Part model, mm, in its own coordinate system. Face numbers are marked on the shaded views. A direction names the side the tool comes from. Give positions to 0.01 mm unless a question says otherwise; leave off trailing zeros. Loops run counter-clockwise (first coordinate to the right, second up) from the corner with the lowest first, then second, coordinate; pieces in that order, holes last. Notation, with made-up numbers: M 43,-12.5 L 59,-12.5 A17 cw 59,10.5 Z; hole C -37.75,17.5 d8. An arc over 180 degrees is marked long. Put each result on its own line as item: value. Start each with the question number.
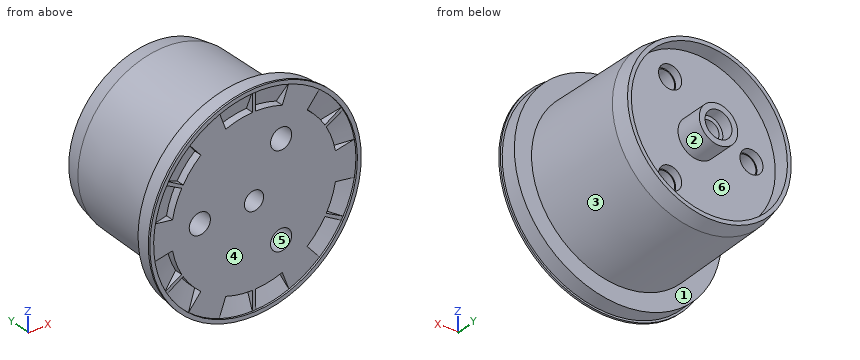
```python
from build123d import *

# Parameters (mm, degrees)
SCHIZZO1_R                    = 22
ESTRUSIONE_ESTRUSIONE1_DEPTH  = 30
SFORMO1_ANGLE                 = 1
SMUSSO1_SIZE                  = 4
SMUSSO1_SIZE2                 = 0.707593191
SCHIZZO2_R                    = 20.292406809
TAGLIO_ESTRUSIONE1_DEPTH      = 4
SCHIZZO4_R                    = 3
TAGLIO_ESTRUSIONE2_DEPTH      = 2
SCHIZZO3_R                    = 5
ESTRUSIONE_ESTRUSIONE2_DEPTH  = 7
SCHIZZO6_R                    = 3.5
TAGLIO_ESTRUSIONE5_DEPTH      = 3
SCHIZZO14_R                   = 27
SCHIZZO14_R_2                 = 22.5
ESTRUSIONE_ESTRUSIONE8_DEPTH  = 4
SCHIZZO16_R                   = 27.5
SCHIZZO16_R_2                 = 26.5
ESTRUSIONE_ESTRUSIONE9_DEPTH  = 0.5
SCHIZZO21_R                   = 22.5
ESTRUSIONE_ESTRUSIONE12_DEPTH = 4
SCHIZZO5_R                    = 2.75
TAGLIO_ESTRUSIONE3_DEPTH      = 49.215661356
RIPETIZIONECIRCOLARE1_COUNT   = 3
SCHIZZO24_R                   = 2.5
TAGLIO_ESTRUSIONE11_DEPTH     = 52.98797938
TAGLIA_RIVOLUZIONE1_ANGLE     = 40
RIVOLUZIONE1_ANGLE            = 2
RIPETIZIONECIRCOLARE2_COUNT   = 6


# Read off the part's stored shape, not the designer's step: Taglia-Rivoluzione1
with BuildPart() as part:
    # Schizzo1 → Estrusione-Estrusione1 (new body)
    with BuildSketch(Plane(origin=(0, 0, 0), x_dir=(1, 0, 0), z_dir=(0, 1, 0))):
        with Locations(Location((0, 0, 0), (0, 0, 270))):
            Circle(SCHIZZO1_R)
    extrude(amount=ESTRUSIONE_ESTRUSIONE1_DEPTH)

    # Sformo1
    sformo1_faces = [part.faces().sort_by_distance(p)[0] for p in [
        (0, 15, -22),
    ]]
    draft(sformo1_faces, Plane.ZX.offset(30), SFORMO1_ANGLE)

    # Smusso1
    smusso1_edges = [part.edges().sort_by_distance(p)[0] for p in [
        (0, 30, -22),
    ]]
    smusso1_side = [part.faces().sort_by_distance(p)[0] for p in [
        (0, 15, -22.261825974),
    ]]
    chamfer(smusso1_edges, length=SMUSSO1_SIZE, length2=SMUSSO1_SIZE2, reference=smusso1_side[0])

    # Schizzo2 → Taglio-Estrusione1 (cut)
    with BuildSketch(Plane(origin=(0, 30, 0), x_dir=(1, 0, 0), z_dir=(0, 1, 0))):
        with Locations(Location((0, 0, 0), (0, 0, 270))):
            Circle(SCHIZZO2_R)
    extrude(amount=-TAGLIO_ESTRUSIONE1_DEPTH, mode=Mode.SUBTRACT)

    # Schizzo4 → Taglio-Estrusione2 (cut)
    with BuildSketch(Plane(origin=(0, 26, 0), x_dir=(1, 0, 0), z_dir=(0, 1, 0))):
        with Locations(Location((7.05, 12.210958193, 0), (0, 0, 270))):
            Circle(SCHIZZO4_R)
    taglio_estrusione2 = extrude(amount=-TAGLIO_ESTRUSIONE2_DEPTH, mode=Mode.SUBTRACT)

    # Schizzo3 → Estrusione-Estrusione2 (add)
    with BuildSketch(Plane(origin=(0, 26, 0), x_dir=(1, 0, 0), z_dir=(0, 1, 0))):
        with Locations(Location((0, 0, 0), (0, 0, 270))):
            Circle(SCHIZZO3_R)
    extrude(amount=ESTRUSIONE_ESTRUSIONE2_DEPTH)

    # Schizzo6 → Taglio-Estrusione5 (cut)
    with BuildSketch(Plane(origin=(0, 33, 0), x_dir=(1, 0, 0), z_dir=(0, 1, 0))):
        with Locations(Location((0, 0, 0), (0, 0, 270))):
            Circle(SCHIZZO6_R)
    extrude(amount=-TAGLIO_ESTRUSIONE5_DEPTH, mode=Mode.SUBTRACT)

    # Schizzo14 → Estrusione-Estrusione8 (add)
    with BuildSketch(Plane.XZ):
        with Locations(Location((0, 0, 0), (0, 0, 270))):
            Circle(SCHIZZO14_R)
        with Locations(Location((0, 0, 0), (0, 0, 270))):
            Circle(SCHIZZO14_R_2, mode=Mode.SUBTRACT)
    extrude(amount=ESTRUSIONE_ESTRUSIONE8_DEPTH)

    # Schizzo16 → Estrusione-Estrusione9 (add)
    with BuildSketch(Plane.XZ.offset(4)):
        with Locations(Location((0, 0, 0), (0, 0, 270))):
            Circle(SCHIZZO16_R)
        with Locations(Location((0, 0, 0), (0, 0, 270))):
            Circle(SCHIZZO16_R_2, mode=Mode.SUBTRACT)
    extrude(amount=ESTRUSIONE_ESTRUSIONE9_DEPTH)

    # Schizzo21 → Estrusione-Estrusione12 (add)
    with BuildSketch(Plane.XZ):
        Circle(SCHIZZO21_R)
    extrude(amount=ESTRUSIONE_ESTRUSIONE12_DEPTH)

    # Schizzo5 → Taglio-Estrusione3 (cut, symmetric)
    with BuildSketch(Plane(origin=(0, 24, 0), x_dir=(1, 0, 0), z_dir=(0, 1, 0))):
        with Locations(Location((7.05, 12.210958193, 0), (0, 0, 270))):
            Circle(SCHIZZO5_R)
    taglio_estrusione3 = extrude(amount=TAGLIO_ESTRUSIONE3_DEPTH, both=True, mode=Mode.SUBTRACT)

    # RipetizioneCircolare1: Taglio-Estrusione2, Taglio-Estrusione3 ×3 about axis
    ripetizionecircolare1_axis = Axis((0, 0, 0), (0, 1, 0))
    add([taglio_estrusione2.rotate(ripetizionecircolare1_axis, i * 360 / RIPETIZIONECIRCOLARE1_COUNT) for i in range(1, RIPETIZIONECIRCOLARE1_COUNT)], mode=Mode.SUBTRACT)
    add([taglio_estrusione3.rotate(ripetizionecircolare1_axis, i * 360 / RIPETIZIONECIRCOLARE1_COUNT) for i in range(1, RIPETIZIONECIRCOLARE1_COUNT)], mode=Mode.SUBTRACT)

    # Schizzo24 → Taglio-Estrusione11 (cut, through all)
    with BuildSketch(Plane(origin=(0, 30, 0), x_dir=(1, 0, 0), z_dir=(0, 1, 0))):
        with Locations(Location((0, 0, 0), (0, 0, 270))):
            Circle(SCHIZZO24_R)
    extrude(amount=-TAGLIO_ESTRUSIONE11_DEPTH, mode=Mode.SUBTRACT)

    # Taglia-Rivoluzione1 outline → Taglia-Rivoluzione1 (revolve, cut)
    with BuildSketch(Plane(origin=(0, 0, 0), x_dir=(0.3420201433256628, 0, -0.9396926207859105), z_dir=(0.9396926207859105, 0, 0.3420201433256628))):
        Polygon((26.5, -4), (21.5, -2), (21.5, -4), align=None)
    taglia_rivoluzione1 = revolve(axis=Axis((0, 0, 0), (0, 1, 0)), revolution_arc=TAGLIA_RIVOLUZIONE1_ANGLE, mode=Mode.SUBTRACT)

    # Schizzo28 → Rivoluzione1 (revolve, symmetric)
    with BuildSketch(Plane(origin=(0, 0, 0), x_dir=(0, 0, -1), z_dir=(1, 0, 0))) as rivoluzione1_sk:
        Polygon((21.5, -4), (21.5, -2), (26.5, -4), align=None)
    rivoluzione1 = revolve(axis=Axis((0, -4.5, 0), (0, 1, 0)), revolution_arc=RIVOLUZIONE1_ANGLE / 2)
    rivoluzione1 = rivoluzione1 + revolve(rivoluzione1_sk.sketch, axis=Axis((0, -4.5, 0), (0, -1, 0)), revolution_arc=RIVOLUZIONE1_ANGLE / 2)

    # RipetizioneCircolare2: Taglia-Rivoluzione1, Rivoluzione1 ×6 about axis
    ripetizionecircolare2_axis = Axis((0, 0, 0), (0, 1, 0))
    add([taglia_rivoluzione1.rotate(ripetizionecircolare2_axis, i * 360 / RIPETIZIONECIRCOLARE2_COUNT) for i in range(1, RIPETIZIONECIRCOLARE2_COUNT)], mode=Mode.SUBTRACT)
    add([rivoluzione1.rotate(ripetizionecircolare2_axis, i * 360 / RIPETIZIONECIRCOLARE2_COUNT) for i in range(1, RIPETIZIONECIRCOLARE2_COUNT)])


solid = part.part
```
1) Band-saw the part on C-C on y = 27. Give the cut face in (x, z).
2) Mould opens along Z. For the marked faces 1, 2 and 3 say: +Z half, -Z half, draft (parallel to the pull), parting line (faces both ways), or undercut.
3) Wall check: L1, parallel to X at y = 29, z = 0; L2, parallel to Z at x = 7, y = 6; L3, parallel to Z at x = 7.5, y = 8. Give the ranges that are in metal, low to high.
4) Which spindle directions (+Z, -Z, +X, -X, +Y, -Y) get a long thin tool onto all of the face, cutting with end or side? Do the marked faces 4, 5 and 6. Say none if no direction does.
5) Band-saw the part on A-A on y = 19. Give the cut face in (x, z) (3 decimals), then the cut area to 3 significant figures.
6) Band-saw the part on B-B on z = 0. State how many separate pieces and enclosed holes the cut face has, then the cut area to 3 significant figures.
7) Band-saw the part on D-D on y = 12.5. Give the cut face in (x, z) (3 decimals), then the cut area to 3 significant figures.
8) Pin check, flat tips, straight feed: pin 1 Ø3 at (x, z) = (17, 18.5) entering from +Y; pin 2 Ø12 at (x, z) = (-10, -5.5) entering from -Y; pin 3 Ø10 at (x, z) = (18.5, -2) entering from +Y. Stop position of each tip, or through.
Evaluation:
1. outline: C 0,0 d43.75; C 0,0 d10; hole C 0,0 d40.58; hole C 0,0 d5
2. face 1: draft
2. face 2: undercut
2. face 3: parting line
3. L1: -21.49 to -20.29, -5 to -2.5, 2.5 to 5, 20.29 to 21.49
3. L2: -21.3 to -14.96, -9.46 to 9.46, 14.96 to 21.3
3. L3: -21.09 to -14.92, -9.5 to 9.5, 14.92 to 21.09
4. face 4: -Y
4. face 5: +Y, -Y
4. face 6: +Y
5. outline: C 0,0 d44.384; hole C -14.1,0 d5.5; hole C 0,0 d5; hole C 7.05,-12.211 d5.5; hole C 7.05,12.211 d5.5
5. area: 1,460 mm2
6. separate pieces: 3
6. enclosed holes: 0
6. area: 1,100 mm2
7. outline: C 0,0 d44.611; hole C -14.1,0 d5.5; hole C 0,0 d5; hole C 7.05,-12.211 d5.5; hole C 7.05,12.211 d5.5
7. area: 1,470 mm2
8. pin 1: y = 0
8. pin 2: y = -4
8. pin 3: y = 30
